Geometry check sheet. Reference: drawing and pictorial views, mm from the part's lowest x, y, z. A direction names the side the tool comes from. Give positions to 0.01 mm unless a question says otherwise; leave off trailing zeros. Write each loop counter-clockwise with the first axis right and the second up, starting at its lowest first coordinate (ties: lowest second). Pieces come first, ordered by that corner, then holes. Notation, with made-up numbers: M -7.5,-32.75 L -2.5,-32.75 A32 cw -2.5,6.25 Z; hole C 60,21 d1. An arc over 180 degrees is marked long. One line per item, written item: value. Start each with the question number.
1. Cross-section at A-A on y = 31. Record the cut outline in (x, z).
2. Release check for a two-part mould opening along Z. For the marked faces 1, 2 and 3 record: pulls with the +Z half, pulls with the -Z half, needs draft (parallel to the pull), parting line crosses it, or undercut.
3. Tool access check on the marked faces 4 and 5. Record the directions out of +Z, -Z, +X, -X, +Y, -Y that give a thin tool (end or side, any length) a straight path to the whole face; none if there is none.
4. Gauge pin test, flat end, axial feed: pin 1 (3 mm diameter, centred on x = 56.5, z = 61.5, fed in from -Y). Record the tip position at first contact, or that the pin passes through.
5. Cross-section at C-C on z = 22.5. Record the cut outline in (x, y).
6. Scan lines: line 1 (X direction, y = 151.55, z = 38.1); line 2 (Z direction, x = 52, y = 144); line 3 (Z direction, x = 38, y = 151). Record each from-to range of solid material in increasing order.
7. Cross-section at B-B on x = 59.5. Record the cut outline in (y, z), then the cut area to 3 significant figures.
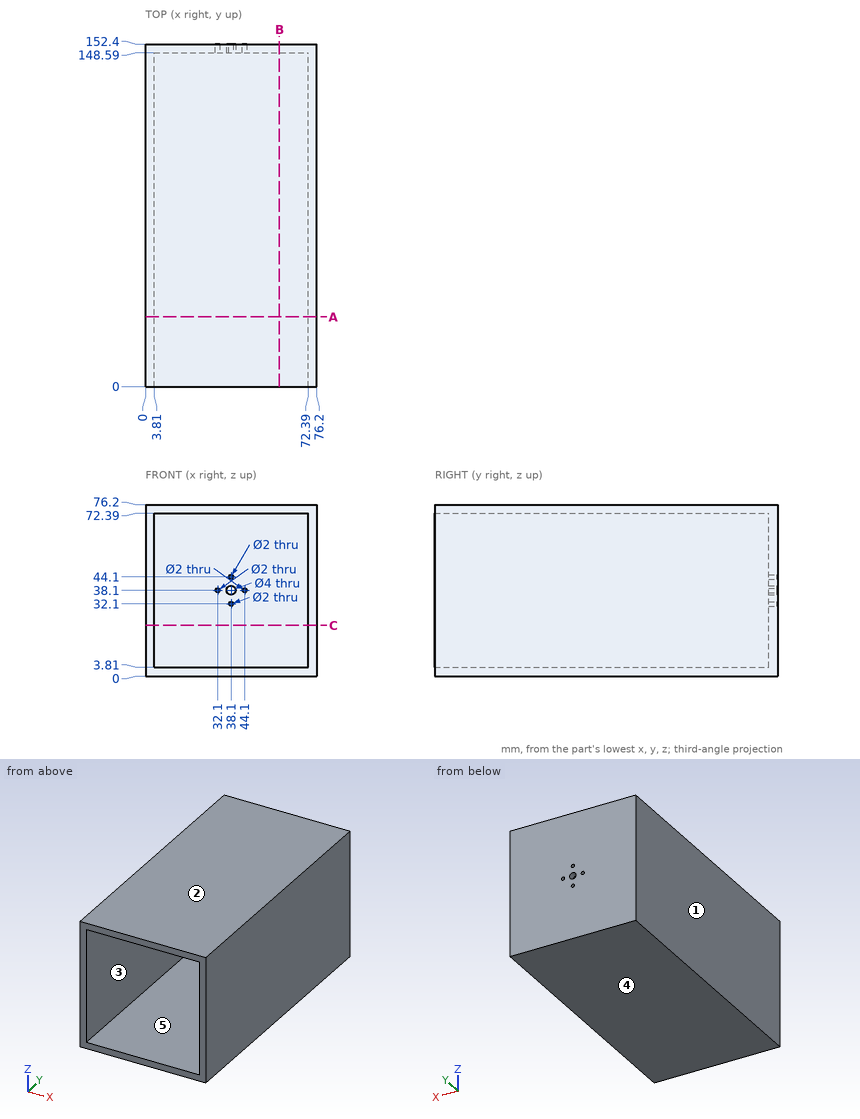
Report:
1. outline: M 0,0 L 76.2,0 L 76.2,76.2 L 0,76.2 Z; hole M 3.81,3.81 L 72.39,3.81 L 72.39,72.39 L 3.81,72.39 Z
2. face 1: needs draft
2. face 2: pulls with the +Z half
2. face 3: undercut
3. face 4: -Z, +X, -X, +Y, -Y
3. face 5: -Y
4. pin 1: stops at y = 148.59
5. outline: M 0,0 L 3.81,0 L 3.81,148.59 L 72.39,148.59 L 72.39,0 L 76.2,0 L 76.2,152.4 L 0,152.4 Z
6. line 1: x = 0 to 31.1, 33.1 to 36.1, 40.1 to 43.1, 45.1 to 76.2
6. line 2: z = 0 to 3.81, 72.39 to 76.2
6. line 3: z = 0 to 31.11, 33.09 to 36.1, 40.1 to 43.11, 45.09 to 76.2
7. outline: M 0,0 L 152.4,0 L 152.4,76.2 L 0,76.2 L 0,72.39 L 148.59,72.39 L 148.59,3.81 L 0,3.81 Z
7. area: 1,420 mm^2
